Can you work these out from the model? Positions are in its coordinate system, mm. A direction names the side the tool comes from. Coordinates: 2 decimals unless noted, no trailing zeros. Order: outer loops, then holes, each group sorted by start corner. A loop starts at its lowest first (then second) coordinate and runs counter-clockwise, first axis right, second up. Notation, with made-up numbers: (-31, 40) - (1, 40) arc R27 cw to (1, 60) - close; hole circle Ø3 at (86, 38.5). An arc over 180 degrees is marked (long way). Use a Markdown table: item, result. Add a question column.
(1) I want a section at A-A (z = 0). List the corners of the cut face in (x, y) for me.
(2) We'd pull the mould along Z, two halves only. Please class faces 1 (the cylindrical face through (-10.2, 15.9, -1.3)), 2 (the flat face through (3, 16.05, 3)), 3 (the cylindrical face through (12.932, 7.395, 5.362)): pulls with the +Z half, pulls with the -Z half, needs draft (parallel to the pull), parting line crosses it, or undercut.
(3) For pin 1 Ø11 at (x, z) = (-7.5, -7.5) entering from +Y; pin 2 Ø2 at (x, y) = (1.5, 2) entering from +Z; pin 3 Ø2 at (y, z) = (9.5, 3.5) entering from +X (3 decimals); pin 4 Ø1 at (y, z) = (10, -10.5) entering from +X, each with a flat end and sliding along its axis, tell me the tip position at first contact or that it passes through.
(4) On a 3-axis mill with a long thin cutter (end or side, diameter ignored), from which of +Z, -Z, +X, -X, +Y, -Y can I reach the whole of each face in a straight line? I mean faces 4 (the flat face through (3, 8, 1.4)), 5 (the cylindrical face through (10.2, 15.9, 1.3)). Say none if no direction works.
(5) I want a section at C-C (x = 0). List the corners of the cut face in (y, z) for me.
(6) If I drill on L1, parallel to X at y = 4, z = -4; L2, parallel to X at y = 7.5, z = -2; L3, parallel to Z at x = -3.5, y = 13, over which ranges is the centre line in solid material (lowest first)? Write a range as [from, to].
(7) I want a section at D-D (z = 7). List the corners of the cut face in (x, y) for me.
(8) I want a section at B-B (y = 1.5). List the corners of the cut face in (x, z) for me.
```python
from build123d import *

# Parameters (mm, degrees)
SKETCH1_R           = 14
BOSS_EXTRUDE2_DEPTH = 16.05
SKETCH3_R           = 14
SKETCH3_R_2         = 12.6
CUT_EXTRUDE1_DEPTH  = 1.05
CUT_EXTRUDE2_DEPTH  = 0.35


with BuildPart() as part:
    # Sketch1 → Boss-Extrude2 (new body)
    with BuildSketch(Plane(origin=(0, 0, 0), x_dir=(1, 0, 0), z_dir=(0, 1, 0))):
        Circle(SKETCH1_R)
        with BuildLine():
            Line((-1.4, 4.2), (-1.4, 2.424871131))
            ThreePointArc((-1.4, 2.424871131), (-1.979898987, 1.979898987), (-2.424871131, 1.4))
            Line((-2.424871131, 1.4), (-4.2, 1.4))
            Line((-4.2, 1.4), (-4.2, -1.4))
            Line((-4.2, -1.4), (-2.424871131, -1.4))
            ThreePointArc((-2.424871131, -1.4), (-1.979898987, -1.979898987), (-1.4, -2.424871131))
            Line((-1.4, -2.424871131), (-1.4, -4.2))
            Line((-1.4, -4.2), (1.4, -4.2))
            Line((1.4, -4.2), (1.4, -2.424871131))
            ThreePointArc((1.4, -2.424871131), (1.979898987, -1.979898987), (2.424871131, -1.4))
            Line((2.424871131, -1.4), (4.2, -1.4))
            Line((4.2, -1.4), (4.2, 1.4))
            Line((4.2, 1.4), (2.424871131, 1.4))
            ThreePointArc((2.424871131, 1.4), (1.979898987, 1.979898987), (1.4, 2.424871131))
            Line((1.4, 2.424871131), (1.4, 4.2))
            Line((1.4, 4.2), (-1.4, 4.2))
        make_face(mode=Mode.SUBTRACT)
    extrude(amount=BOSS_EXTRUDE2_DEPTH)

    # Sketch3 → Cut-Extrude1 (cut)
    with BuildSketch(Plane(origin=(0, 16.05, 0), x_dir=(1, 0, 0), z_dir=(0, 1, 0))):
        Circle(SKETCH3_R)
        Circle(SKETCH3_R_2, mode=Mode.SUBTRACT)
    extrude(amount=-CUT_EXTRUDE1_DEPTH, mode=Mode.SUBTRACT)

    # Sketch3_3 → Cut-Extrude2 (cut)
    with BuildSketch(Plane(origin=(0, 16.05, 0), x_dir=(1, 0, 0), z_dir=(0, 1, 0))):
        with BuildLine():
            ThreePointArc((-3.004809746, 11.152292069), (-8.167083323, 8.167083323), (-11.152292069, 3.004809746))
            ThreePointArc((-11.152292069, 3.004809746), (-10.164718454, 1.288797405), (-8.448706113, 2.27637102))
            ThreePointArc((-8.448706113, 2.27637102), (-6.187184335, 6.187184335), (-2.27637102, 8.448706113))
            ThreePointArc((-2.27637102, 8.448706113), (-1.288797405, 10.164718454), (-3.004809746, 11.152292069))
        make_face()
        with BuildLine():
            ThreePointArc((-11.152292069, -3.004809746), (-8.167083323, -8.167083323), (-3.004809746, -11.152292069))
            ThreePointArc((-3.004809746, -11.152292069), (-1.288797405, -10.164718454), (-2.27637102, -8.448706113))
            ThreePointArc((-2.27637102, -8.448706113), (-6.187184335, -6.187184335), (-8.448706113, -2.27637102))
            ThreePointArc((-8.448706113, -2.27637102), (-10.164718454, -1.288797405), (-11.152292069, -3.004809746))
        make_face()
        with BuildLine():
            ThreePointArc((3.004809746, -11.152292069), (8.167083323, -8.167083323), (11.152292069, -3.004809746))
            ThreePointArc((11.152292069, -3.004809746), (10.164718454, -1.288797405), (8.448706113, -2.27637102))
            ThreePointArc((8.448706113, -2.27637102), (6.187184335, -6.187184335), (2.27637102, -8.448706113))
            ThreePointArc((2.27637102, -8.448706113), (1.288797405, -10.164718454), (3.004809746, -11.152292069))
        make_face()
        with BuildLine():
            ThreePointArc((11.152292069, 3.004809746), (8.167083323, 8.167083323), (3.004809746, 11.152292069))
            ThreePointArc((3.004809746, 11.152292069), (1.288797405, 10.164718454), (2.27637102, 8.448706113))
            ThreePointArc((2.27637102, 8.448706113), (6.187184335, 6.187184335), (8.448706113, 2.27637102))
            ThreePointArc((8.448706113, 2.27637102), (10.164718454, 1.288797405), (11.152292069, 3.004809746))
        make_face()
    extrude(amount=-CUT_EXTRUDE2_DEPTH, mode=Mode.SUBTRACT)


solid = part.part
```
Answers follow:
| question | item | result |
|---|---|---|
| 1 | outline | (-14, 0) - (-4.2, 0) - (-4.2, 16.05) - (-12.6, 16.05) - (-12.6, 15) - (-14, 15) - close; (4.2, 0) - (14, 0) - (14, 15) - (12.6, 15) - (12.6, 16.05) - (4.2, 16.05) - close |
| 2 | face 1 | undercut |
| 2 | face 2 | needs draft |
| 2 | face 3 | parting line crosses it |
| 3 | pin 1 | stops at y = 16.05 |
| 3 | pin 2 | stops at z = 13.99 |
| 3 | pin 3 | stops at x = 13.775 |
| 3 | pin 4 | stops at x = 9.8 |
| 4 | face 4 | +Y, -Y |
| 4 | face 5 | +Y |
| 5 | outline | (0, -14) - (15, -14) - (15, -12.6) - (16.05, -12.6) - (16.05, -4.2) - (0, -4.2) - close; (0, 4.2) - (16.05, 4.2) - (16.05, 12.6) - (15, 12.6) - (15, 14) - (0, 14) - close |
| 6 | L1 | x = [-13.42, -1.4], [1.4, 13.42] |
| 6 | L2 | x = [-13.86, -1.96], [1.96, 13.86] |
| 6 | L3 | z = [-13.56, -1.4], [1.4, 13.56] |
| 7 | outline | (-12.12, 0) - (12.12, 0) - (12.12, 15) - (10.48, 15) - (10.48, 16.05) - (9.19, 16.05) - (9.19, 15.7) - (5.25, 15.7) - (5.25, 16.05) - (-5.25, 16.05) - (-5.25, 15.7) - (-9.19, 15.7) - (-9.19, 16.05) - (-10.48, 16.05) - (-10.48, 15) - (-12.12, 15) - close |
| 8 | outline | circle Ø28 at (0, 0); hole (-4.2, -1.4) - (-2.42, -1.4) arc R2.8 ccw to (-1.4, -2.42) - (-1.4, -4.2) - (1.4, -4.2) - (1.4, -2.42) arc R2.8 ccw to (2.42, -1.4) - (4.2, -1.4) - (4.2, 1.4) - (2.42, 1.4) arc R2.8 ccw to (1.4, 2.42) - (1.4, 4.2) - (-1.4, 4.2) - (-1.4, 2.42) arc R2.8 ccw to (-2.42, 1.4) - (-4.2, 1.4) - close |
